For this review, take the finished solid that the model builds, in its own axes (mm). A direction names the side the tool comes from. Coordinates: 2 decimals unless noted, no trailing zeros. Write each loop counter-clockwise with the first axis right and the second up, starting at its lowest first coordinate (ties: lowest second). Pieces come first, ordered by that corner, then holes. Notation, with made-up numbers: M 76.5,87 L 81.5,87 A22 cw 81.5,119 Z; hole C 67.25,-3 d2. An arc over 180 degrees is marked long. One line per question, with ' | ' between items.
from build123d import *

# Parameters (mm, degrees)
SKETCH1_W           = 50
SKETCH1_H           = 70
BOSS_EXTRUDE1_DEPTH = 50
SKETCH2_R           = 15
BOSS_EXTRUDE2_DEPTH = 10
SKETCH3_R           = 4
BOSS_EXTRUDE3_DEPTH = 5
SHELL7_START        = 2
SHELL7_OUTLINE_W    = 46
SHELL7_OUTLINE_H    = 66
SHELL7_DEPTH        = 46
SHELL7_START_2      = 48
SHELL7_2_OUTLINE_R  = 13
SHELL7_2_DEPTH      = 10
SHELL7_START_3      = 58
SHELL7_3_OUTLINE_R  = 2
SHELL7_3_DEPTH      = 5
SKETCH4_R           = 4
BOSS_EXTRUDE4_DEPTH = 5


# Read off the part's stored shape, not the designer's step: Shell7
with BuildPart() as part:
    # Sketch1 → Boss-Extrude1 (new body)
    with BuildSketch(Plane(origin=(0, 0, 0), x_dir=(1, 0, 0), z_dir=(0, 1, 0))):
        with Locations((25, 35)):
            Rectangle(SKETCH1_W, SKETCH1_H)
    extrude(amount=BOSS_EXTRUDE1_DEPTH)

    # Sketch2 → Boss-Extrude2 (add)
    with BuildSketch(Plane(origin=(0, 50, 0), x_dir=(1, 0, 0), z_dir=(0, 1, 0))):
        with Locations(Location((20, 20, 0), (0, 0, 90))):
            Circle(SKETCH2_R)
    extrude(amount=BOSS_EXTRUDE2_DEPTH)

    # Sketch3 → Boss-Extrude3 (add)
    with BuildSketch(Plane(origin=(0, 60, 0), x_dir=(1, 0, 0), z_dir=(0, 1, 0))):
        with Locations(Location((20, 20, 0), (0, 0, 270))):
            Circle(SKETCH3_R)
    extrude(amount=BOSS_EXTRUDE3_DEPTH)

    # Shell7 outline → Shell7 (cut)
    with BuildSketch(Plane(origin=(0, 0, 0), x_dir=(1, 0, 0), z_dir=(0, 1, 0)).offset(SHELL7_START)):
        with Locations((25, 35)):
            Rectangle(SHELL7_OUTLINE_W, SHELL7_OUTLINE_H)
    extrude(amount=SHELL7_DEPTH, mode=Mode.SUBTRACT)

    # Shell7 2 outline → Shell7 2 (cut)
    with BuildSketch(Plane(origin=(0, 0, 0), x_dir=(1, 0, 0), z_dir=(0, 1, 0)).offset(SHELL7_START_2)):
        with Locations((20, 20)):
            Circle(SHELL7_2_OUTLINE_R)
    extrude(amount=SHELL7_2_DEPTH, mode=Mode.SUBTRACT)

    # Shell7 3 outline → Shell7 3 (cut)
    with BuildSketch(Plane(origin=(0, 0, 0), x_dir=(1, 0, 0), z_dir=(0, 1, 0)).offset(SHELL7_START_3)):
        with Locations((20, 20)):
            Circle(SHELL7_3_OUTLINE_R)
    extrude(amount=SHELL7_3_DEPTH, mode=Mode.SUBTRACT)

    # Sketch4 → Boss-Extrude4 (add)
    with BuildSketch(Plane(origin=(0, 50, 0), x_dir=(1, 0, 0), z_dir=(0, 1, 0))):
        with BuildLine():
            Line((17.5, 70), (32.5, 70))
            Line((32.5, 70), (32.5, 80))
            ThreePointArc((32.5, 80), (25, 87.5), (17.5, 80))
            Line((17.5, 80), (17.5, 70))
        make_face()
        with Locations(Location((25, 80, 0), (0, 0, 270))):
            Circle(SKETCH4_R, mode=Mode.SUBTRACT)
    boss_extrude4 = extrude(amount=-BOSS_EXTRUDE4_DEPTH)

    # Mirror1: Boss-Extrude4 across plane
    add(boss_extrude4.mirror(Plane(origin=(0, 0, -35), x_dir=(1, 0, 0), z_dir=(0, 0, -1))))


solid = part.part
1) The part is to be moulded in two halves that separate along Z. For faces 1 (the cylindrical face through (23.966, 62.465, -20.521)), 2 (the flat face through (50, 25, -35)), 3 (the flat face through (25, 2, -35)), 4 (the cylindrical face through (32.4, 52.9, -23.9)), say which applies: +Z half, -Z half, draft (parallel to the pull), parting line (faces both ways), or undercut.
Responses:
face 1: parting line | face 2: draft | face 3: undercut | face 4: undercut
2) Insertion check: pin 1 Ø1.5 at (y, z) = (47.5, -77) entering from -X; pin 2 Ø14 at (x, y) = (20.5, 16) entering from +Z; pin 3 Ø5.5 at (y, z) = (48.5, -77) entering from +X. Each pin has a flat end and moves straight along its axis. Give the tip position at first contact, or say it passes through.
Responses:
pin 1: x = 17.5 | pin 2: z = 0 | pin 3: x = 32.5
3) Machinability: for faces 5 (the flat face through (17.5, 48, -75)), 6 (the flat face through (23, 58, -20)), 7 (the flat face through (32.5, 48, -75)), 8 (the flat face through (23, 60, -23)), which of the approach directions +Z, -Z, +X, -X, +Y, -Y give a long, thin tool a straight path to every point of the face, cutting with its end or side? Answer none if there is none.
Responses:
face 5: -Z, -X, +Y, -Y | face 6: none | face 7: -Z, +X, +Y, -Y | face 8: +Y
4) We need section B-B on y = 20. State the section outline as (x, z) points.
Responses:
outline: M 0,-70 L 50,-70 L 50,0 L 0,0 Z; hole M 2,-68 L 48,-68 L 48,-2 L 2,-2 Z
5) We need section D-D on z = -9.5. State the section outline as (x, y) points, then the cut area to 3 significant figures.
Responses:
outline: M 0,0 L 50,0 L 50,50 L 30.71,50 L 30.71,60 L 9.29,60 L 9.29,50 L 0,50 Z; hole M 2,2 L 48,2 L 48,48 L 27.66,48 L 27.66,58 L 12.34,58 L 12.34,48 L 2,48 Z | area: 445 mm^2
6) We need section C-C on z = -20. State the section outline as (x, y) points.
Responses:
outline: M 0,0 L 50,0 L 50,50 L 35,50 L 35,60 L 24,60 L 24,65 L 16,65 L 16,60 L 5,60 L 5,50 L 0,50 Z; hole M 2,2 L 48,2 L 48,48 L 33,48 L 33,58 L 22,58 L 22,63 L 18,63 L 18,58 L 7,58 L 7,48 L 2,48 Z
7) To check wall thickness, follow line 1 along Y through (x, z) = (29.5, -6); line 2 along X through (y, z) = (49, 10); line 3 along X through (y, z) = (50.75, -20). State the ranges of each line that lie inside material, in increasing order. Write a range as [from, to].
Responses:
line 1: [0, 2], [48, 50] | line 2: [17.5, 21], [29, 32.5] | line 3: [5, 7], [33, 35]
8) We need section A-A on z = -59. State the section outline as (x, y) points, then the cut area to 3 significant figures.
Responses:
outline: M 0,0 L 50,0 L 50,50 L 0,50 Z; hole M 2,2 L 48,2 L 48,48 L 2,48 Z | area: 384 mm^2
